The figure shows three views and two pictorial views of one solid part (mm, origin at its lowest corner). Answer the questions. Give positions to 0.01 mm unless a question says otherwise; leave off trailing zeros. Order: outer loops, then holes, each group sorted by start corner. A loop starts at its lowest first (then second) coordinate and runs counter-clockwise, first axis right, second up. Notation, with made-up numbers: M 41,51.5 L 74,51.5 A9 ccw 74,55.5 Z; hole C 2,-13 d4. An arc over 180 degrees is marked long. Answer as a JSON object with one key per item and string values. Group by question number.
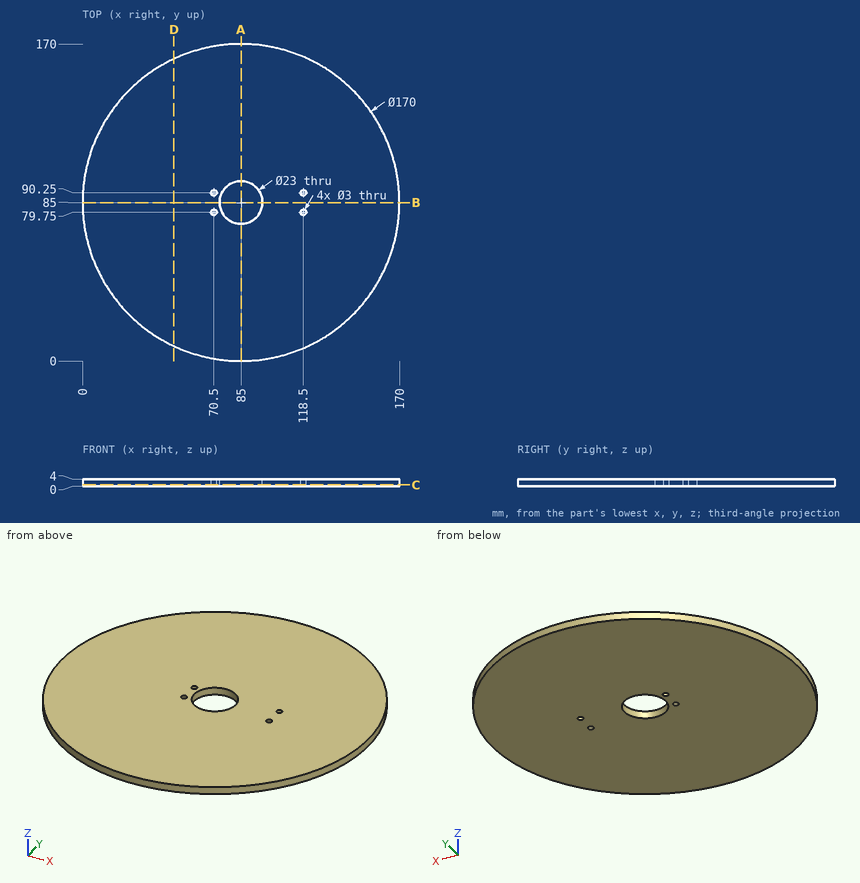
Item 1: Section D-D (x = 49) is taken. Determine the outline of the cut face in (y, z).
Item 2: Section C-C (z = 0.8) is taken. Determine the outline of the cut face in (x, y), and give its area (3 significant figures).
Item 3: Consider probe 1 along Y at (x, z) = (70.5, 2.5); probe 2 along Y at (x, z) = (118.5, 3.1); probe 3 along Y at (x, z) = (85, 1.4). Determine where each line is inside the solid, lowest interval first. Write a range as from..to.
Item 4: Flat-ended cylindrical pins translate along their axes: P1, Ø2, axis at x = 79.5, z = 2.5, coming from the +Y side; P2, Ø1.5, axis at y = 81.5, z = 3, coming from the -X side; P3, Ø4, axis at x = 118.5, y = 79.75, coming from the -Z side; P4, Ø1, axis at x = 31.5, z = 1.5, coming from the +Y side. Find the tip coordinate at first contact, or state that the pin passes through.
Item 5: Section A-A (x = 85) is taken. Determine the outline of the cut face in (y, z).
Values found:
{
 "1": {"outline": "M 8,0 L 162,0 L 162,4 L 8,4 Z"},
 "2": {"outline": "C 85,85 d170; hole C 70.5,79.75 d3; hole C 70.5,90.25 d3; hole C 85,85 d23; hole C 118.5,79.75 d3; hole C 118.5,90.25 d3", "area": "22,300 mm^2"},
 "3": {"probe 1": "y = 1.25..78.25, 81.25..88.75, 91.75..168.75", "probe 2": "y = 6.88..78.25, 81.25..88.75, 91.75..163.12", "probe 3": "y = 0..73.5, 96.5..170"},
 "4": {"P1": "stops at y = 169.88", "P2": "stops at x = 0.04", "P3": "stops at z = 0", "P4": "stops at y = 151.45"},
 "5": {"outline": "M 0,0 L 73.5,0 L 73.5,4 L 0,4 Z; M 96.5,0 L 170,0 L 170,4 L 96.5,4 Z"}
}
